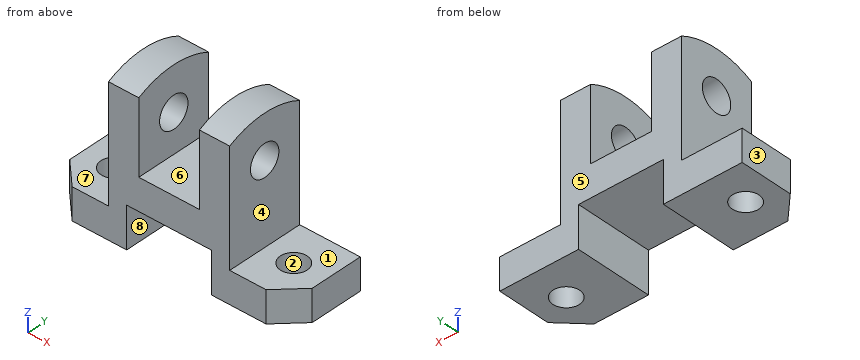
```python
from build123d import *

# Parameters (mm, degrees)
F1_DEPTH = 50
F2_W     = 35
F2_H     = 17
F2_W_2   = 25
F2_H_2   = 40.236561
F2_H_3   = 60.406679
F3_DEPTH = 32.001
F4_R     = 5.5
F5_DEPTH = 13.001
F6_R     = 5.5
F7_DEPTH = 13.001
F8_R     = 6.5
F9_DEPTH = 75.001


with BuildPart() as f1:
    # F0 (on Right) → F1 (new body, symmetric)
    with BuildSketch(Plane.YZ):
        with BuildLine():
            Line((-16, 60.128765), (-16, 0))
            Line((-16, 0), (16, 0))
            Line((16, 0), (16, 60.128765))
            ThreePointArc((16, 60.128765), (0, 64), (-16, 60.128765))
        make_face()
    extrude(amount=F1_DEPTH, both=True)

    # F2 (on face) → F3 (cut, through all)
    with BuildSketch(Plane.XZ.offset(16)):
        with Locations((0, 8.5)):
            Rectangle(F2_W, F2_H)
        with Locations((0, 50.11828)):
            Rectangle(F2_W_2, F2_H_2)
        with Locations((-37.5, 43.203339)):
            Rectangle(F2_W_2, F2_H_3)
        with Locations((37.5, 43.203339)):
            Rectangle(F2_W_2, F2_H_3)
    extrude(amount=-F3_DEPTH, mode=Mode.SUBTRACT)

    # F4 (on face) → F5 (cut, through all)
    with BuildSketch(Plane.XY.offset(13)):
        Polygon((-40, -16), (-50, -6), (-50, -16), align=None)
        with Locations((-37, 0)):
            Circle(F4_R)
    extrude(amount=-F5_DEPTH, mode=Mode.SUBTRACT)

    # F6 (on face) → F7 (cut, through all)
    with BuildSketch(Plane.XY.offset(13)):
        Polygon((50, -6), (40, -16), (50, -16), align=None)
        with Locations((37, 0)):
            Circle(F6_R)
    extrude(amount=-F7_DEPTH, mode=Mode.SUBTRACT)

    # F8 (on face) → F9 (cut, through all)
    with BuildSketch(Plane.YZ.offset(25)):
        with Locations((0, 46)):
            Circle(F8_R)
    extrude(amount=-F9_DEPTH, mode=Mode.SUBTRACT)


solid = f1.part
```
Part model, mm, in its own coordinate system. Face numbers are marked on the shaded views. A direction names the side the tool comes from. Round coordinates to 2 decimals unless told otherwise and drop trailing zeros. Write each loop counter-clockwise with the first axis right and the second up, starting at its lowest first coordinate (ties: lowest second). Pieces come first, ordered by that corner, then holes. Notation, with made-up numbers: (84.25, 54.25) -> (117.25, 54.25) arc R18 cw to (117.25, 77.25) -> close; hole circle Ø9 at (39.25, 78.5). An arc over 180 degrees is marked (long way). Return JSON: item names as keys, results as strings. Group by question number.
Q1. Saw through at B-B on z = 46. Write the cut outline in (x, y), plus the area to 3 significant figures.
Q2. Saw through at C-C on y = 0. State how many separate pieces and enclosed holes the cut face has, plus the area to 3 significant figures.
Q3. Which spindle directions (+Z, -Z, +X, -X, +Y, -Y) get a long thin tool onto all of the face, cutting with end or side? Do the marked faces 4, 5, 6, 7 and 8. Say none if no direction does.
Q4. Probe L1, parallel to Z at x = -19, y = 0; L2, parallel to X at y = -11.5, z = 45.5; L3, parallel to X at y = 6, z = 7. List the from-to ranges inside material, lowest first. Write a range as [from, to].
Q5. Pin check, flat tips, straight feed: pin 1 (16 mm diameter, centred on x = -3.5, y = 4.5, fed in from -Z); pin 2 (17.5 mm diameter, centred on x = 37, y = 0, fed in from +Z); pin 3 (1 mm diameter, centred on x = -10.5, z = 42.5, fed in from +Y); pin 4 (15 mm diameter, centred on y = 0, z = 46, fed in from -X). Stop position of each tip, or through.
Q6. Saw through at A-A on z = 58. Write the cut outline in (x, y), plus the area to 3 significant figures.
Q7. Saw through at D-D on x = -37. Write the cut outline in (y, z), plus the area to 3 significant figures.
Q8. Mould opens along X. For the marked faces 1, 2 and 3 say: pulls with the +X half, pulls with the -X half, needs draft (parallel to the pull), parting line crosses it, or undercut.
Answer:
{
 "1": {"outline": "(-25, -16) -> (-12.5, -16) -> (-12.5, -6.5) -> (-25, -6.5) -> close; (-25, 6.5) -> (-12.5, 6.5) -> (-12.5, 16) -> (-25, 16) -> close; (12.5, -16) -> (25, -16) -> (25, -6.5) -> (12.5, -6.5) -> close; (12.5, 6.5) -> (25, 6.5) -> (25, 16) -> (12.5, 16) -> close", "area": "475 mm2"},
 "2": {"separate pieces": "5", "enclosed holes": "0", "area": "1,790 mm2"},
 "3": {"face 4": "+Z, +X, +Y, -Y", "face 5": "+Z, -Z, +X, -X, +Y", "face 6": "+Z, +Y, -Y", "face 7": "+Z, -X, +Y, -Y", "face 8": "-Z, +Y, -Y"},
 "4": {"L1": "[0, 39.5], [52.5, 64]", "L2": "[-25, -12.5], [12.5, 25]", "L3": "[-50, -17.5], [17.5, 50]"},
 "5": {"pin 1": "z = 17", "pin 2": "z = 13", "pin 3": "through", "pin 4": "x = -25"},
 "6": {"outline": "(-25, -16) -> (-12.5, -16) -> (-12.5, 16) -> (-25, 16) -> close; (12.5, -16) -> (25, -16) -> (25, 16) -> (12.5, 16) -> close", "area": "800 mm2"},
 "7": {"outline": "(-16, 0) -> (-5.5, 0) -> (-5.5, 13) -> (-16, 13) -> close; (5.5, 0) -> (16, 0) -> (16, 13) -> (5.5, 13) -> close", "area": "273 mm2"},
 "8": {"face 1": "needs draft", "face 2": "undercut", "face 3": "pulls with the -X half"}
}
